```python
from build123d import *

# Parameters (mm, degrees)
F0_R     = 61.5
F0_R_2   = 2.1
F0_R_3   = 51.5
F1_DEPTH = 2.5


with BuildPart() as f1:
    # F0 (on Top) → F1 (new body, symmetric)
    with BuildSketch(Plane.XY):
        Circle(F0_R)
        with Locations((-28.1, -48.670628)):
            Circle(F0_R_2, mode=Mode.SUBTRACT)
        with Locations((-52.810725, -19.221532)):
            Circle(F0_R_2, mode=Mode.SUBTRACT)
        with Locations((9.759028, -55.346196)):
            Circle(F0_R_2, mode=Mode.SUBTRACT)
        with Locations((43.051698, -36.124664)):
            Circle(F0_R_2, mode=Mode.SUBTRACT)
        with Locations((-52.810725, 19.221532)):
            Circle(F0_R_2, mode=Mode.SUBTRACT)
        with Locations((-28.1, 48.670628)):
            Circle(F0_R_2, mode=Mode.SUBTRACT)
        Circle(F0_R_3, mode=Mode.SUBTRACT)
        with Locations((56.2, 0)):
            Circle(F0_R_2, mode=Mode.SUBTRACT)
        with Locations((9.759028, 55.346196)):
            Circle(F0_R_2, mode=Mode.SUBTRACT)
        with Locations((43.051698, 36.124664)):
            Circle(F0_R_2, mode=Mode.SUBTRACT)
    extrude(amount=F1_DEPTH, both=True)


solid = f1.part
```
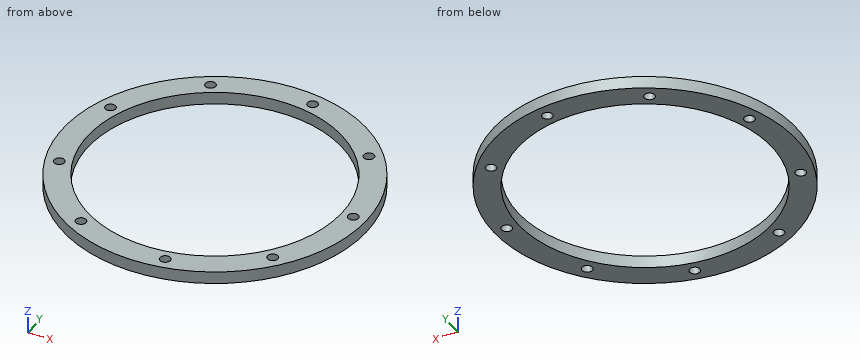
Geometry check sheet. Reference: the model listing, model coordinates, mm. Coordinates: 2 decimals unless noted, no trailing zeros. Order: outer loops, then holes, each group sorted by start corner. A loop starts at its lowest first (then second) coordinate and runs counter-clockwise, first axis right, second up. Notation, with made-up numbers: (78, 59) - (97, 59) arc R32 cw to (97, 85) - close; hole circle Ø9 at (28, 61). An arc over 180 degrees is marked (long way). Answer as a JSON object with one key per item and string values. Group by question number.
Item 1: Scan lines: probe 1 along Y at (x, z) = (0, -0.1); probe 2 along X at (y, z) = (-28.5, 0.45); probe 3 along X at (y, z) = (8, -0.7). Record each from-to range of solid material in increasing order.
Item 2: Sectioned sample at C-C, the plane y = 44. Record the cut outline in (x, z).
Item 3: Depth check by flat-ended pin: pin 1 Ø3.5 at (x, y) = (9.76, 55.35) entering from +Z; pin 2 Ø1 at (x, z) = (-26.5, -0.5) entering from -Y; pin 3 Ø3 at (y, z) = (29.5, -1.5) entering from -X; pin 4 Ø1 at (x, z) = (45.5, 1.5) entering from +Y. Enter the tip coordinate at first touch or a pass-through.
Item 4: Sectioned sample at A-A, the plane x = 0. Record the cut outline in (y, z).
Item 5: Sectioned sample at D-D, the plane x = -53. Record the cut outline in (y, z).
Item 6: Sectioned sample at B-B, the plane y = 0. Record the cut outline in (x, z).
Resolved:
{
 "1": {"probe 1": "-61.5 to -51.5, 51.5 to 61.5", "probe 2": "-54.5 to -42.9, 42.9 to 54.5", "probe 3": "-60.98 to -50.87, 50.87 to 60.98"},
 "2": {"outline": "(-42.97, -2.5) - (-26.76, -2.5) - (-26.76, 2.5) - (-42.97, 2.5) - close; (26.76, -2.5) - (42.97, -2.5) - (42.97, 2.5) - (26.76, 2.5) - close"},
 "3": {"pin 1": "through", "pin 2": "y = -55.73", "pin 3": "x = -54.76", "pin 4": "y = 41.92"},
 "4": {"outline": "(-61.5, -2.5) - (-51.5, -2.5) - (-51.5, 2.5) - (-61.5, 2.5) - close; (51.5, -2.5) - (61.5, -2.5) - (61.5, 2.5) - (51.5, 2.5) - close"},
 "5": {"outline": "(-31.2, -2.5) - (-21.31, -2.5) - (-21.31, 2.5) - (-31.2, 2.5) - close; (-17.13, -2.5) - (17.13, -2.5) - (17.13, 2.5) - (-17.13, 2.5) - close; (21.31, -2.5) - (31.2, -2.5) - (31.2, 2.5) - (21.31, 2.5) - close"},
 "6": {"outline": "(-61.5, -2.5) - (-51.5, -2.5) - (-51.5, 2.5) - (-61.5, 2.5) - close; (51.5, -2.5) - (54.1, -2.5) - (54.1, 2.5) - (51.5, 2.5) - close; (58.3, -2.5) - (61.5, -2.5) - (61.5, 2.5) - (58.3, 2.5) - close"}
}
